Job drawing, mm, ordinate dimensions from the low corner. One solid piece. A direction names the side the tool comes from. Round coordinates to 2 decimals unless told otherwise and drop trailing zeros. Order: outer loops, then holes, each group sorted by start corner. A loop starts at its lowest first (then second) coordinate and runs counter-clockwise, first axis right, second up. Notation, with made-up numbers: (23.25, 37) -> (41.25, 37) arc R30 ccw to (41.25, 64) -> close; hole circle Ø2 at (23, 85.5). An arc over 180 degrees is marked (long way). Answer as a JSON object with one key per item and string values. Group by question number.
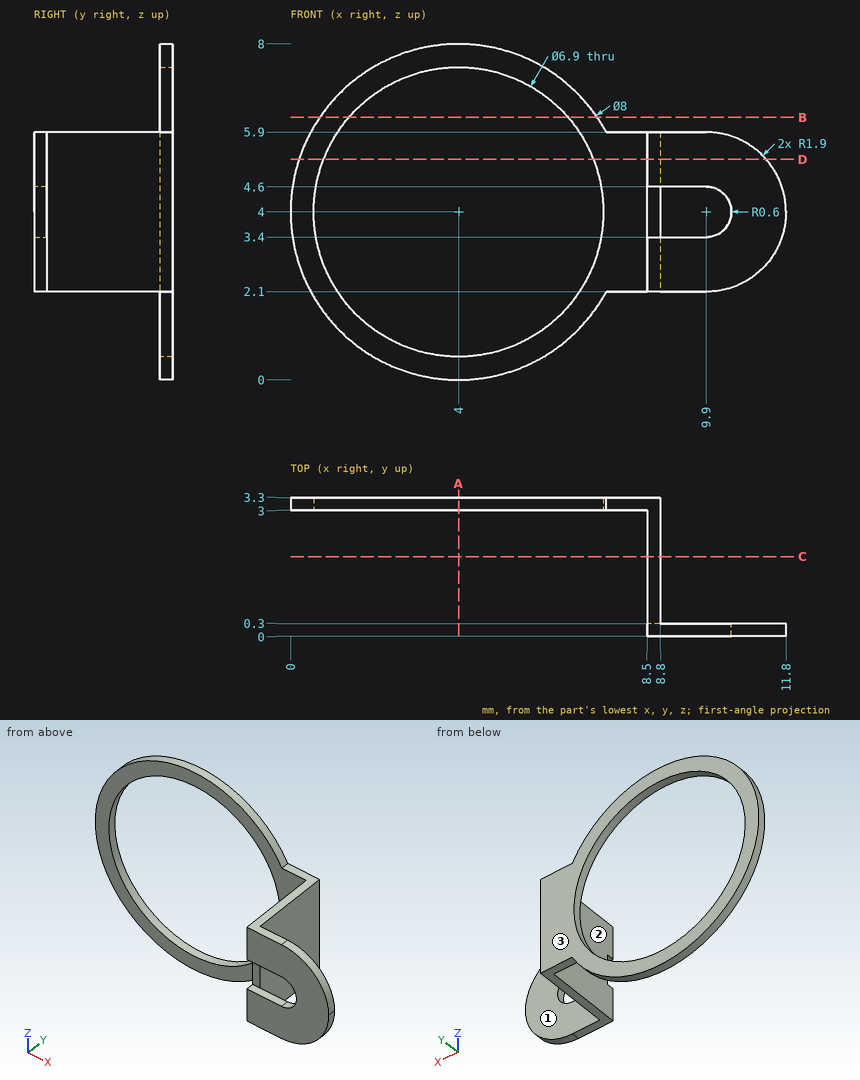
Q1. Drop flat-ended pins along their axis: pin 1 Ø1.5 at (y, z) = (0.5, 2) entering from +X; pin 2 Ø1.5 at (x, z) = (11, 4.5) entering from +Y; pin 3 Ø0.9 at (y, z) = (1.5, 3) entering from -X. Give the stop position or say it passes through.
Q2. Wall check: line 1 (X direction, y = 3.1, z = 4); line 2 (X direction, y = 0.75, z = 3); line 3 (Y direction, x = 10.5, z = 4.25). Give the ranges that are in metal, low to high. Write a range as [from, to].
Q3. Band-saw the part on C-C (y = 1.9). List the corners of the cut face in (x, z).
Q4. Band-saw the part on D-D (z = 5.25). List the corners of the cut face in (x, y), plus the area to 3 significant figures.
Q5. Which spindle directions (+Z, -Z, +X, -X, +Y, -Y) get a long thin tool onto all of the face, cutting with end or side? Do the marked faces 1, 2 and 3. Say none if no direction does.
Q6. Band-saw the part on B-B (z = 6.25). List the corners of the cut face in (x, y).
Q7. Band-saw the part on A-A (x = 4). List the corners of the cut face in (y, z).
Completed:
{
 "1": {"pin 1": "x = 11.31", "pin 2": "y = 0.3", "pin 3": "x = 8.5"},
 "2": {"line 1": "[0, 0.55], [7.45, 8.8]", "line 2": "[8.5, 8.8]", "line 3": "[0, 0.3]"},
 "3": {"outline": "(8.5, 2.1) -> (8.8, 2.1) -> (8.8, 5.9) -> (8.5, 5.9) -> close"},
 "4": {"outline": "(0.2, 3) -> (0.78, 3) -> (0.78, 3.3) -> (0.2, 3.3) -> close; (7.22, 3) -> (8.5, 3) -> (8.5, 0) -> (11.33, 0) -> (11.33, 0.3) -> (8.8, 0.3) -> (8.8, 3.3) -> (7.22, 3.3) -> close", "area": "2.31 mm2"},
 "5": {"face 1": "+Z, -Z, +X, +Y", "face 2": "+Z, -Z, -X, -Y", "face 3": "+Z, -Z, +X, -X, +Y"},
 "6": {"outline": "(0.69, 3) -> (1.38, 3) -> (1.38, 3.3) -> (0.69, 3.3) -> close; (6.62, 3) -> (7.31, 3) -> (7.31, 3.3) -> (6.62, 3.3) -> close"},
 "7": {"outline": "(3, 0) -> (3.3, 0) -> (3.3, 0.55) -> (3, 0.55) -> close; (3, 7.45) -> (3.3, 7.45) -> (3.3, 8) -> (3, 8) -> close"}
}
